Could you check a few things on this model? Use its own coordinates, in mm. Face numbers are marked on the shaded views. Give positions to 0.01 mm unless a question says otherwise; leave off trailing zeros. Loops run counter-clockwise (first coordinate to the right, second up) from the corner with the lowest first, then second, coordinate; pieces in that order, holes last. Notation, with made-up numbers: (77.5, 60.5) -> (104.5, 60.5) arc R29 cw to (104.5, 96.5) -> close; hole circle Ø4 at (58.25, 47.5). An arc over 180 degrees is marked (long way). Write item = value, one per line. Start each with the question number.
1) I want a section at A-A (y = 8). List the corners of the cut face in (x, z) for me.
2) I'm going to push a flat-ended pin straight in: pin 1 Ø3 at (x, y) = (0.48, 17.29) entering from +Z. Where does the tip first touch, or does it pass through?
3) I need wall thicknesses on probe 1 along Y at (x, z) = (0.75, 1.5); probe 2 along X at (y, z) = (17.5, 2.6); probe 3 along Y at (x, z) = (17.75, 1.25). Which ranges of each line are inside material? Lowest first, please. Write a range as from..to.
4) If we mould it in two halves opening along Y, with no side actions, what happens to the marked faces 1, 2 and 3? For each: +Y half, -Y half, draft (parallel to the pull), parting line (faces both ways), or undercut.
5) I want a section at B-B (z = 0.65). Count the separate pieces of the cut face and the enclosed holes in it, and give its area (3 significant figures).
6) I want a section at C-C (x = 11). List the corners of the cut face in (y, z) for me.
7) I want a section at D-D (y = 2). List the corners of the cut face in (x, z) for me, and give its area (3 significant figures).
from build123d import *

# Parameters (mm, degrees)
SKETCH_1_R          = 1.35
SKETCH_1_R_2        = 1.3
EXTRUDE_1_DEPTH     = 3
SKETCH_2_R          = 1.6
CUT_EXTRUDE_1_DEPTH = 40.58429055


with BuildPart() as part:
    # 草图1 → 凸台-拉伸1 (new body)
    with BuildSketch(Plane(origin=(0, 0, 0), x_dir=(-1, 0, 0), z_dir=(0, 0, -1))):
        with BuildLine():
            Line((3.311115848, 16.021732214), (3.313115848, 16.021732214))
            ThreePointArc((3.313115848, 16.021732214), (1.422584465, 20.809546819), (-3.619383376, 19.772320768))
            ThreePointArc((-3.619383376, 19.772320768), (-3.907451025, 19.356483629), (-4.140741668, 18.907619539))
            ThreePointArc((-4.140741668, 18.907619539), (-9.493299368, 12.888445888), (-17.351741668, 11.120619539))
            ThreePointArc((-17.351741668, 11.120619539), (-19.703460244, 10.604408599), (-21.333741668, 8.832619539))
            ThreePointArc((-21.333741668, 8.832619539), (-21.651545732, 6.446374123), (-20.542741668, 4.309619539))
            ThreePointArc((-20.542741668, 4.309619539), (-9.614805592, -11.161234041), (-4.459741668, -29.387380461))
            ThreePointArc((-4.459741668, -29.387380461), (-3.626617209, -31.434284825), (-1.833741668, -32.726380461))
            ThreePointArc((-1.833741668, -32.726380461), (0.370527809, -32.871130249), (2.315258332, -31.823380461))
            ThreePointArc((2.315258332, -31.823380461), (3.407459975, -29.901725556), (3.313258332, -27.693380461))
            ThreePointArc((3.313258332, -27.693380461), (-0.247316641, -5.861423686), (3.295002421, 15.973502613))
            Line((3.295002421, 15.973502613), (3.311115848, 16.021732214))
        make_face()
        with Locations(Location((-17.711384152, 7.136232214, 0), (0, 0, 180))):
            Circle(SKETCH_1_R, mode=Mode.SUBTRACT)
        with Locations(Location((-0.480884152, -28.962767786, 0), (0, 0, 180))):
            Circle(SKETCH_1_R_2, mode=Mode.SUBTRACT)
        with Locations(Location((-0.480884152, 17.291232214, 0), (0, 0, 180))):
            Circle(SKETCH_1_R_2, mode=Mode.SUBTRACT)
    extrude(amount=-EXTRUDE_1_DEPTH)

    # 草图2 → 切除-拉伸1 (cut, through all)
    with BuildSketch(Plane.XY.offset(3)):
        with Locations((0.480884152, 17.291232214)):
            Circle(SKETCH_2_R)
        with Locations((17.711384152, 7.136232214)):
            Circle(SKETCH_2_R)
    extrude(amount=-CUT_EXTRUDE_1_DEPTH, mode=Mode.SUBTRACT)


solid = part.part
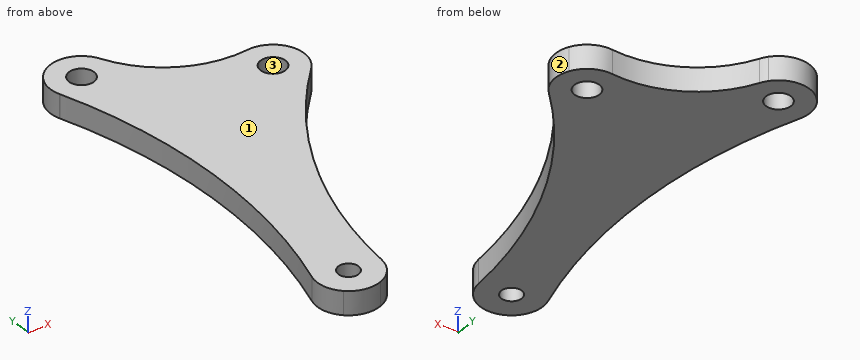
Answer list:
q1.outline = (-1.16, 0) -> (16.36, 0) -> (16.36, 3) -> (-1.16, 3) -> close; (19.06, 0) -> (21.62, 0) -> (21.62, 3) -> (19.06, 3) -> close
q2.pin_1 = through
q3.probe_1 = -32.95..-30.23, -27.69..15.71, 18.87..21.28
q3.probe_2 = -3.51..-1.11, 2.07..4.87
q3.probe_3 = 1.3..5.54, 8.74..11.14
q4.face_1 = draft
q4.face_2 = parting line
q4.face_3 = undercut
q5.separate_pieces = 1
q5.enclosed_holes = 3
q5.area = 612 mm^2
q6.outline = (-8.45, 0) -> (12.13, 0) -> (12.13, 3) -> (-8.45, 3) -> close
q7.outline = (-0.2, 0) -> (18.36, 0) -> (18.36, 3) -> (-0.2, 3) -> close
q7.area = 55.7 mm^2
